Part model, mm, in its own coordinate system. Face numbers are marked on the shaded views. Give positions to 0.01 mm unless a question says otherwise; leave off trailing zeros. Write each loop counter-clockwise with the first axis right and the second up, starting at its lowest first coordinate (ties: lowest second). Pieces come first, ordered by that corner, then holes.
Autodesk Inventor part; units mm, degrees
ref_plane "YZ Plane" through (0, 0, 0) normal (1, 0, 0) x (0, 1, 0)
ref_plane "XZ Plane" through (0, 0, 0) normal (0, 1, 0) x (-1, 0, 0)
ref_plane "XY Plane" through (0, 0, 0) normal (0, 0, 1) x (1, 0, 0)
sketch "Sketch1" plane through (0, 0, 0) normal (0, 0, 1) x (1, 0, 0)
  line L0 (-8.76, 11.0126) -> (-8.76, 0.5126)
  line L1 (-8.76, 0.5126) -> (-11.24, -14.9874)
  line L2 (-11.24, -14.9874) -> (8.76, -14.9874)
  line L3 (8.76, -14.9874) -> (8.76, -4.4874)
  line L4 (11.24, 11.0126) -> (-8.76, 11.0126)
  line L5 (0, 12.916) -> (0, -18.5653)
  line L6 (-8.76, 0.5126) -> (13.6474, 0.5126) construction
  line L7 (8.76, -4.4874) -> (-2.6872, -4.4874) construction
  line L8 (-5.8361, -1.9874) -> (18.6079, -1.9874) construction
  circle A0 centre (0, -7.7374) radius 1.325
  circle A1 centre (0, 3.7626) radius 1.325
  line L9 (22.7948, -1.9874) -> (0, -1.9874) construction
  line L10 (9.36, -0.7374) -> (0, -0.7374)
  line L11 (0, -3.2374) -> (8.96, -3.2374)
  arc A2 (0, -0.7374) -> (0, -3.2374) centre (0, -1.9874) ccw
  line L12 (8.76, -4.4874) -> (8.96, -3.2374)
  line L13 (9.36, -0.7374) -> (11.24, 11.0126)
  point P0 (0, 0)
  point P1 (-8.76, -4.4874)
  point P2 (11.3974, -1.9874)
  dimension "d0" = 2.48
  dimension "d1" = 15.5
  dimension "d2" = 15.5
  dimension "d3" = 2.48
  dimension "d4" = 10.5
  dimension "d5" = 10.5
  dimension "d6" = 20
  dimension "d7" = 20
  dimension "d8" = 2.65
  dimension "d9" = 7.25
  dimension "d12" = 2.5
  dimension "d26" = 11.75
  dimension "d27" = 14.25
extrude "Extrusion1" add sketch "Sketch1" against normal blind 2.8 contours L4 L5 A1 A2 A0 L2 L1 L0 | L4 L13 L10 L5 A1 | L5 A0 L11 L12 L3 L2
sketch "Sketch2" plane through (0, 0, 0) normal (0, 0, 1) x (1, 0, 0)
  line L0 (-67.25, -18.5874) -> (-67.25, 14.6126)
  line L1 (0, 12.916) -> (0, -18.5653) construction
  line L2 (-5.8361, -1.9874) -> (18.6079, -1.9874) construction
  line L3 (-67.25, 14.6126) -> (-67.25, 18.4126)
  line L4 (-57.4847, 14.6126) -> (-57.4847, 17.8301)
  arc A0 (-57.4847, 17.8301) -> (-67.25, 18.4126) centre (-62.35, 18.4126) ccw
  line L5 (0, 12.916) -> (0, -18.5653)
  circle A1 centre (-62.35, 18.4126) radius 2.1
  arc A2 (0, -0.7374) -> (0, -3.2374) centre (0, -1.9874) ccw
  line L6 (-1.25, -1.9874) -> (17.7749, -1.9874) construction
  line L7 (0, -3.2374) -> (67.25, -3.2374)
  line L8 (67.25, -0.7374) -> (0, -0.7374)
  arc A3 (0, -0.7374) -> (0, -3.2374) centre (0, -1.9874) ccw
  line L9 (67.25, 14.6126) -> (67.25, -0.7374)
  line L10 (67.25, -3.2374) -> (67.25, -18.5874)
  line L11 (-4.9, -18.5874) -> (-24.8081, -18.5874)
  circle A4 centre (0, 3.7626) radius 1.325
  circle A5 centre (0, -7.7374) radius 1.325
  line L12 (67.25, 14.6126) -> (67.25, 18.4126)
  line L13 (57.4847, 14.6126) -> (57.4847, 17.8301)
  arc A6 (67.25, 18.4126) -> (57.4847, 17.8301) centre (62.35, 18.4126) ccw
  circle A7 centre (62.35, 18.4126) radius 2.1
  line L14 (-67.25, -18.5874) -> (-67.25, -22.3874)
  line L15 (-57.4847, -18.5874) -> (-57.4847, -21.8049)
  arc A8 (-67.25, -22.3874) -> (-57.4847, -21.8049) centre (-62.35, -22.3874) ccw
  circle A9 centre (-62.35, -22.3874) radius 2.1
  line L16 (57.4847, -18.5874) -> (57.4847, -21.8049)
  circle A10 centre (62.35, -22.3874) radius 2.1
  line L17 (67.25, -18.5874) -> (67.25, -22.3874)
  arc A11 (57.4847, -21.8049) -> (67.25, -22.3874) centre (62.35, -22.3874) ccw
  line L18 (-4.9, 14.6126) -> (-4.9, 18.4126)
  line L19 (4.8653, 14.6126) -> (4.8653, 17.8301)
  arc A12 (4.8653, 17.8301) -> (-4.9, 18.4126) centre (0, 18.4126) ccw
  circle A13 centre (0, 18.4126) radius 2.1
  line L20 (-57.4847, 14.6126) -> (-4.9, 14.6126)
  line L21 (4.8653, 14.6126) -> (57.4847, 14.6126)
  line L22 (-4.9, -18.5874) -> (-4.9, -22.3874)
  line L23 (4.8653, -18.5874) -> (4.8653, -21.8049)
  arc A14 (-4.9, -22.3874) -> (4.8653, -21.8049) centre (0, -22.3874) ccw
  circle A15 centre (0, -22.3874) radius 2.1
  line L24 (57.4847, -18.5874) -> (4.8653, -18.5874)
  line L25 (-4.9, -18.5874) -> (-57.4847, -18.5874)
  point P0 (0, 0)
  point P1 (8.2624, -1.9874)
  point P2 (67.25, 14.6126)
  point P3 (39.75, 14.6126)
  point P4 (67.25, -18.5874)
  dimension "d15" = 4.9
  dimension "d16" = 4.2
  dimension "d25" = 134.5
  dimension "d38" = 4.9
  dimension "d39" = 4.2
extrude "Extrusion2" add sketch "Sketch2" along normal blind 2.75 contours L0 L3 A0 L4 L20 L18 A12 L19 L21 L13 A6 L12 L9 L8 A2 L7 L10 L17 A11 L16 L24 L23 A14 L22 L11 L25 L15 A8 L14
sketch "Sketch3" plane through (0, 0, 2.75) normal (0, 0, 1) x (1, 0, 0)
  arc A0 (0, -0.7374) -> (0, -3.2374) centre (0, -1.9874) ccw
  line L0 (0, -1.9874) -> (79.0333, -1.9874) construction
  line L1 (0, -5.2374) -> (79.0333, -5.2374)
  line L2 (79.0333, 1.2626) -> (0, 1.2626)
  arc A1 (0, 1.2626) -> (0, -5.2374) centre (0, -1.9874) ccw
  arc A2 (79.0333, -5.2374) -> (79.0333, 1.2626) centre (79.0333, -1.9874) ccw
  point P0 (0, 0)
  point P1 (39.5166, -1.9874)
  dimension "d20" = 3.25
extrude "Extrusion3" cut sketch "Sketch3" against normal blind 1.65
sketch "Sketch4" plane through (0, 0, 0) normal (0, 0, -1) x (-1, 0, 0)
  line L0 (-62.15, 8.0126) -> (-60.65, 8.0126)
  line L1 (-60.65, 8.0126) -> (-60.65, -0.7874)
  line L2 (-60.65, -0.7874) -> (-62.15, -0.7874)
  line L3 (-62.15, -0.7874) -> (-62.15, 8.0126)
  line L4 (-67.25, -0.7374) -> (-67.25, 18.4126)
  line L5 (-57.4847, 14.6126) -> (57.4847, 14.6126)
  line L6 (60.65, -3.1874) -> (62.15, -3.1874)
  line L7 (62.15, -3.1874) -> (62.15, -11.9874)
  line L8 (62.15, -11.9874) -> (60.65, -11.9874)
  line L9 (60.65, -11.9874) -> (60.65, -3.1874)
  line L10 (67.25, 18.4126) -> (67.25, -22.3874)
  line L11 (57.4847, -18.5874) -> (-57.4847, -18.5874)
  point P0 (0, 0)
  point P1 (-67.25, 8.8376)
  dimension "d28" = 5.1
  dimension "d29" = 6.6
  dimension "d30" = 8.8
  dimension "d31" = 1.5
  dimension "d32" = 5.1
  dimension "d34" = 8.8
  dimension "d35" = 1.5
extrude "Extrusion4" add sketch "Sketch4" along normal blind 2.3
properties part number "Gripper_BackPlate_Long"
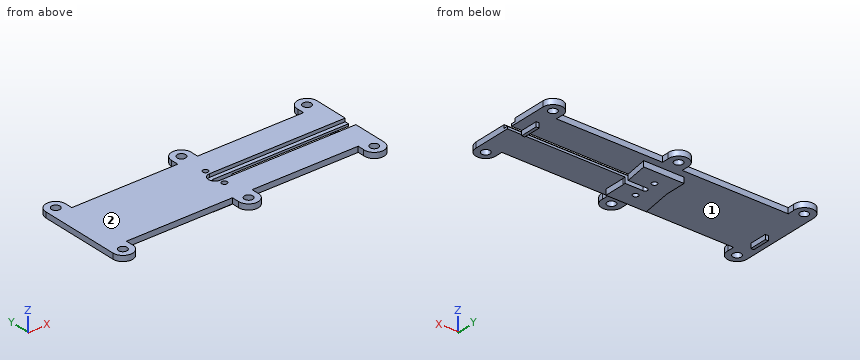
1) Saw through at B-B, the plane x = 41. Write the cut outline in (y, z).
Answers follow:
outline: (-18.59, 0) - (-3.24, 0) - (-3.24, 1.1) - (-5.24, 1.1) - (-5.24, 2.75) - (-18.59, 2.75) - close; (-0.74, 0) - (14.61, 0) - (14.61, 2.75) - (1.26, 2.75) - (1.26, 1.1) - (-0.74, 1.1) - close
2) Saw through at A-A, the plane z = -1.4. Write the cut outline in (x, y) (3 decimals), then the cut area to 3 significant figures.
Answers follow:
outline: (-62.15, -11.987) - (-60.65, -11.987) - (-60.65, -3.187) - (-62.15, -3.187) - close; (-11.24, -14.987) - (8.76, -14.987) - (8.76, -4.487) - (8.96, -3.237) - (0, -3.237) arc R1.25 cw to (0, -0.737) - (9.36, -0.737) - (11.24, 11.013) - (-8.76, 11.013) - (-8.76, 0.513) - close; (60.65, -0.787) - (62.15, -0.787) - (62.15, 8.013) - (60.65, 8.013) - close; hole circle Ø2.65 at (0, -7.737); hole circle Ø2.65 at (0, 3.763)
area: 484 mm2
3) Saw through at C-C, the plane x = -15. Write the cut outline in (y, z).
Answers follow:
outline: (-18.59, 0) - (14.61, 0) - (14.61, 2.75) - (-18.59, 2.75) - close
4) Two-plate mould, pull along X, no slides. Class the marked faces 1 and 2: +X half, -X half, draft (parallel to the pull), parting line (faces both ways), or undercut.
Answers follow:
face 1: undercut
face 2: draft
5) Wall check: L1, parallel to X at y = 15, z = 1.1; L2, parallel to Y at x = 0, z = -1.25; L3, parallel to Y at x = 62.35, z = 2.05. Give the ranges that are in metal, low to high.
Answers follow:
L1: x = -67.25 to -57.48, -4.9 to 4.87, 57.48 to 67.25
L2: y = -14.99 to -9.06, -6.41 to -3.24, -0.74 to 2.44, 5.09 to 11.01
L3: y = -27.29 to -24.49, -20.29 to -5.24, 1.26 to 16.31, 20.51 to 23.31
6) Pin check, flat tips, straight feed: pin 1 Ø1.4 at (x, z) = (-39, 1.5) entering from +Y; pin 2 Ø1.6 at (x, y) = (-61.5, -8) entering from -Z; pin 3 Ø1.2 at (y, z) = (-9, -1.5) entering from +X; pin 4 Ø3 at (y, z) = (17, -2) entering from -X. Stop position of each tip, or through.
Answers follow:
pin 1: stops at y = 14.61
pin 2: stops at z = -2.3
pin 3: stops at x = 8.76
pin 4: passes through
